```python
from build123d import *

# Parameters (mm, degrees)
F0_W     = 75
F0_H     = 50
F1_DEPTH = 1374
F3_DEPTH = 50.001


with BuildPart() as f1:
    # F0 (on Front) → F1 (new body, symmetric)
    with BuildSketch(Plane.XZ):
        with Locations((37.5, 25)):
            Rectangle(F0_W, F0_H)
    extrude(amount=F1_DEPTH, both=True)

    # F2 (on face) → F3 (cut, through all)
    with BuildSketch(Plane.XY.offset(50)):
        Polygon((0, 1374), (75, 1299), (75, 1374), align=None)
        Polygon((0, -1374), (75, -1374), (0, -1299), align=None)
    extrude(amount=-F3_DEPTH, mode=Mode.SUBTRACT)

    # F5: sweep along a path in F5_path
    with BuildLine(Plane(origin=(75, 1299, 0), x_dir=(0.7071067812, -0.7071067812, 0), z_dir=(0.7071067812, 0.7071067812, 0))) as f5_path:
        Line((0, 0), (-106.066017178, 0))
    # F4 (on face) → F5 (sweep, cut)
    with BuildSketch(Plane(origin=(0, 0, 0), x_dir=(0, -1, 0), z_dir=(-1, 0, 0))):
        Polygon((-1333.5107983402, 0), (-1374, 50), (-1374, 0), align=None)
    sweep(path=f5_path.line, mode=Mode.SUBTRACT)


solid = f1.part
```
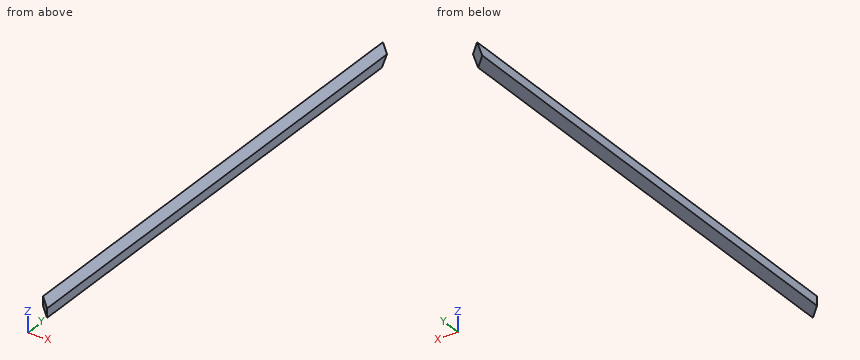
Geometry check sheet. Reference: the model listing, model coordinates, mm. Give positions to 0.01 mm unless a question says otherwise; leave off trailing zeros. Order: outer loops, then holes, each group sorted by start corner. A loop starts at its lowest first (then second) coordinate and runs counter-clockwise, first axis right, second up.
1. Section check A-A, the plane x = 47.5. Enter the section's corners in (y, z), and give its area (3 significant figures).
2. Thickness scan on L1, parallel to Y at x = 47, z = 28; L2, parallel to Y at x = 69.5, z = 23. Record the ranges inside material, lowest first.
3. Section check B-B, the plane z = 14.5. Enter the section's corners in (x, y).
4. Gauge pin test, flat ends, axial feed: pin 1 Ø8 at (x, z) = (22, 23) entering from +Y; pin 2 Ø3 at (x, z) = (54.5, 18) entering from -Y. Record the tip position at first contact, or that the pin passes through.
Values follow:
1. outline: (-1346.5, 0) - (1286.01, 0) - (1326.5, 50) - (-1346.5, 50) - close
1. area: 133,000 mm2
2. L1: y = -1346 to 1309.18
2. L2: y = -1368.5 to 1282.64
3. outline: (0, -1299) - (75, -1374) - (75, 1270.25) - (0, 1345.25) - close
4. pin 1: stops at y = 1335.28
4. pin 2: stops at y = -1355
